Could you check a few things on this drawing? It's one solid part, dimensions in mm from its lowest x, y, z. A direction names the side the tool comes from. Round coordinates to 2 decimals unless told otherwise and drop trailing zeros. Write each loop counter-clockwise with the first axis right and the second up, starting at its lowest first coordinate (ties: lowest second). Pieces come first, ordered by that corner, then holes. Notation, with made-up numbers: (-15.75, 35) - (19.25, 35) arc R19 cw to (19.25, 41) - close; hole circle Ø10 at (60.5, 70.25). An arc over 180 degrees is marked (long way). Write item = value, one per line. Start each with the question number.
Item 1: If we section it at A-A (z = 1.5): Please give me the cut outline in (x, y), and give its area (3 significant figures).
Item 2: If I drill on line 1 along Y through (x, z) = (3, 2.6); line 2 along X through (y, z) = (3.5, 3.6); line 3 along Z through (x, y) = (18.25, 4.75), over which ranges is the centre line in solid material (lowest first)? Write a range as [from, to].
Item 3: Thinking about a two-plate mould opening in X: for the marked faces 1, 2 and 3, which applies, pulls with the +X half, pulls with the -X half, needs draft (parallel to the pull), parting line crosses it, or undercut?
Item 4: Which directions (+Z, -Z, +X, -X, +Y, -Y) give clear straight access to the entire face, cutting with the end or side of a thin tool? Please do the marked faces 4, 5 and 6.
Item 5: For P1, Ø2.5, axis at x = 16, y = 3, coming from the +Z side; P2, Ø1.5, axis at y = 1.5, z = 3, coming from the -X side, each with a flat end and sliding along its axis, tell me the tip position at first contact or that it passes through.
Item 6: If we section it at B-B (x = 16.25): Please give me the cut outline in (y, z).
Item 7: If we section it at C-C (z = 3.5): Please give me the cut outline in (x, y).
Item 8: If we section it at D-D (y = 1): Please give me the cut outline in (x, z), and give its area (3 significant figures).
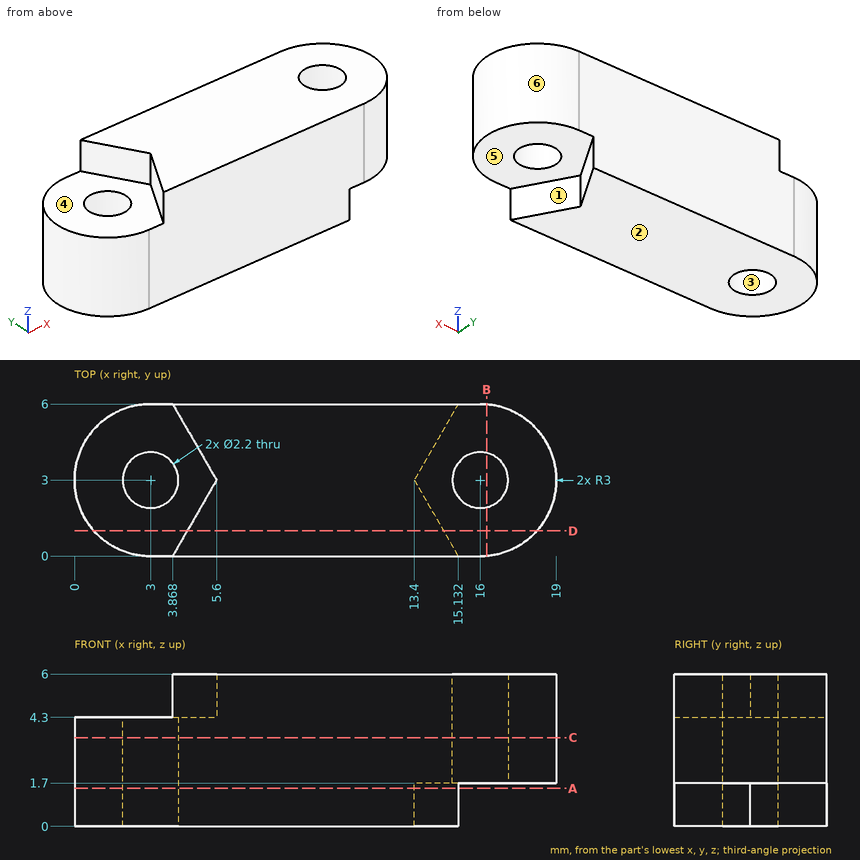
Reply:
q1.outline = (3, 0) - (15.13, 0) - (13.4, 3) - (15.13, 6) - (3, 6) arc R3 ccw to start; hole circle Ø2.2 at (3, 3)
q1.area = 77.9 mm2
q2.line_1 = [0, 1.9], [4.1, 6]
q2.line_2 = [0.04, 2.02], [3.98, 15.02], [16.98, 18.96]
q2.line_3 = [1.7, 6]
q3.face_1 = pulls with the +X half
q3.face_2 = needs draft
q3.face_3 = undercut
q4.face_4 = +Z, -X
q4.face_5 = -Z, +X
q4.face_6 = +Z, -Z, +X
q5.P1 = 6
q5.P2 = 0.1
q6.outline = (0.01, 1.7) - (1.93, 1.7) - (1.93, 6) - (0.01, 6) - close; (4.07, 1.7) - (5.99, 1.7) - (5.99, 6) - (4.07, 6) - close
q7.outline = (3, 0) - (16, 0) arc R3 ccw to (16, 6) - (3, 6) arc R3 ccw to start; hole circle Ø2.2 at (3, 3); hole circle Ø2.2 at (16, 3)
q8.outline = (0.76, 0) - (14.55, 0) - (14.55, 1.7) - (18.24, 1.7) - (18.24, 6) - (4.45, 6) - (4.45, 4.3) - (0.76, 4.3) - close
q8.area = 92.3 mm2
